Verification items for the finished model (mm, model axes). Coordinates: 2 decimals unless noted, no trailing zeros. Write each loop counter-clockwise with the first axis right and the second up, starting at its lowest first coordinate (ties: lowest second). Pieces come first, ordered by that corner, then holes. Notation, with made-up numbers: M 29.25,0 L 88.25,0 A25 cw 88.25,24 Z; hole C 45.25,-32 d4. An arc over 180 degrees is marked long. One line per item, written item: value.
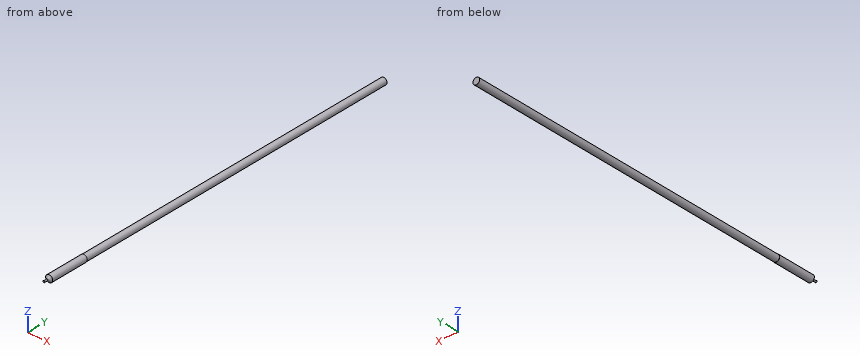
```python
from build123d import *


with BuildPart() as part:
    # Sketch2 → Revolve1 (revolve)
    with BuildSketch(Plane(origin=(0, 0, 0), x_dir=(0, 0, -1), z_dir=(1, 0, 0)), mode=Mode.PRIVATE) as revolve1_sk:
        with BuildLine():
            Line((0.925, -4.438709677), (0.925, 5.95))
            Line((0.925, 5.95), (0.875, 5.95))
            Line((0.875, 5.95), (0.875, 95.95))
            Line((0.875, 95.95), (0, 95.95))
            Line((0, 95.95), (0, -6.1))
            ThreePointArc((0, -6.1), (0.13462912, -6.0740728), (0.25, -6))
            Line((0.25, -6), (0.2, -6))
            Line((0.2, -6), (0.2, -5))
            Line((0.2, -5), (0.925, -4.438709677))
        make_face()
    revolve(revolve1_sk.sketch.rotate(Axis((0, 105.424070968, 0), (0, -1, 0)), 180), axis=Axis((0, 105.424070968, 0), (0, -1, 0)))


solid = part.part
```
Item 1: Cross-section at B-B, the plane y = 4. Enter the section's corners in (x, z) (3 decimals), and give its area (3 significant figures).
The answers:
outline: C 0,0 d1.85
area: 2.69 mm²
Item 2: Scan lines: line 1 (X direction, y = 8, z = 0.1); line 2 (Y direction, x = -0.1, z = 0.4); line 3 (Z direction, x = 0.1, y = 2). Record each from-to range of solid material in increasing order.
The answers:
line 1: x = -0.87 to 0.87
line 2: y = -4.84 to 95.95
line 3: z = -0.92 to 0.92
Item 3: Cross-section at A-A, the plane y = 63. Enter the section's corners in (x, z) (3 decimals).
The answers:
outline: C 0,0 d1.75
